```python
from build123d import *

# Parameters (mm, degrees)
F1_DEPTH = 1.5875
F2_R     = 3.175
F3_DEPTH = 3.176


with BuildPart() as f1:
    # F0 (on Top) → F1 (new body, symmetric)
    with BuildSketch(Plane.XY):
        Polygon((76.2, -31.2657933708), (76.2, 31.2657933708), (31.5991683182, 76.4655258179), (-31.9008316818, 75.9372385012), (-76.2, 31.4872385012), (-76.2, -32.5658159349), (-29.7164364601, -77.0158159349), (32.6911213348, -75.3589100367), align=None)
    extrude(amount=F1_DEPTH, both=True)

    # F2 (on face) → F3 (cut, through all)
    with BuildSketch(Plane.XY.offset(1.5875)):
        with Locations((-66.675, 6.35)):
            Circle(F2_R)
        with Locations((-66.675, -6.35)):
            Circle(F2_R)
        with Locations((6.35, -66.5299041307)):
            Circle(F2_R)
        with Locations((-6.35, -66.8670861268)):
            Circle(F2_R)
        with Locations((66.675, -6.35)):
            Circle(F2_R)
        with Locations((66.675, 6.35)):
            Circle(F2_R)
        with Locations((6.35, 66.730136108)):
            Circle(F2_R)
        with Locations((-6.35, 66.6244786446)):
            Circle(F2_R)
    extrude(amount=-F3_DEPTH, mode=Mode.SUBTRACT)


solid = f1.part
```
Check sheet for the modelled part. Datum: model origin and axes. Units: mm. Round coordinates to 2 decimals unless told otherwise and drop trailing zeros. Write each loop counter-clockwise with the first axis right and the second up, starting at its lowest first coordinate (ties: lowest second). Pieces come first, ordered by that corner, then holes. Notation, with made-up numbers: (-29.75, -5.5) -> (0.25, -5.5) arc R34 cw to (0.25, 28.5) -> close; hole circle Ø8 at (46.25, 57). An arc over 180 degrees is marked (long way). Put each result on its own line as item: value.
(1) Go/stop test with flat-tipped pins: pin 1 Ø1 at (x, z) = (36.5, 0) entering from +Y; pin 2 Ø1.5 at (y, z) = (53.5, -1) entering from +X; pin 3 Ø1 at (y, z) = (61, 1) entering from +X. Record where each tip stops, or that it passes through.
Values found:
pin 1: stops at y = 72.01
pin 2: stops at x = 55
pin 3: stops at x = 47.35
(2) Material ranges on line 1 (X direction, y = 6.5, z = 0.35); line 2 (Y direction, x = -6.35, z = -0.15); line 3 (X direction, y = -65, z = 0.65), recorded low to high.
Values found:
line 1: x = -76.2 to -69.85, -63.5 to 63.5, 69.85 to 76.2
line 2: y = -76.4 to -70.04, -63.69 to 63.45, 69.8 to 76.15
line 3: x = -42.28 to -8.92, -3.78 to 3.57, 9.13 to 42.91
(3) Sectioned sample at A-A (y = -6.35). Enter the section's corners in (x, z).
Values found:
outline: (-76.2, -1.59) -> (-69.85, -1.59) -> (-69.85, 1.59) -> (-76.2, 1.59) -> close; (-63.5, -1.59) -> (63.5, -1.59) -> (63.5, 1.59) -> (-63.5, 1.59) -> close; (69.85, -1.59) -> (76.2, -1.59) -> (76.2, 1.59) -> (69.85, 1.59) -> close
(4) Sectioned sample at B-B (x = 5.5). Enter the section's corners in (y, z).
Values found:
outline: (-76.08, -1.59) -> (-69.59, -1.59) -> (-69.59, 1.59) -> (-76.08, 1.59) -> close; (-63.47, -1.59) -> (63.67, -1.59) -> (63.67, 1.59) -> (-63.47, 1.59) -> close; (69.79, -1.59) -> (76.25, -1.59) -> (76.25, 1.59) -> (69.79, 1.59) -> close
(5) Sectioned sample at C-C (z = -0.2). Count the separate pieces of the cut face and the enclosed holes in it, plus the area to 3 significant figures.
Values found:
separate pieces: 1
enclosed holes: 8
area: 19,000 mm^2
(6) Mould release check, pull along Y, two halves, no side actions. Record for faces 1 (the face through (-1, 1, -1.588)), 2 (the face through (-64.97, 9.03, 0.02)), 3 (the face through (-53.284, -54.48, 0.022)): released by +Y, released by -Y, zero draft, split by the parting line, or undercut.
Values found:
face 1: zero draft
face 2: undercut
face 3: released by -Y
(7) Sectioned sample at D-D (y = -45). Enter the section's corners in (x, z), plus the area to 3 significant figures.
Values found:
outline: (-63.2, -1.59) -> (62.65, -1.59) -> (62.65, 1.59) -> (-63.2, 1.59) -> close
area: 400 mm^2
